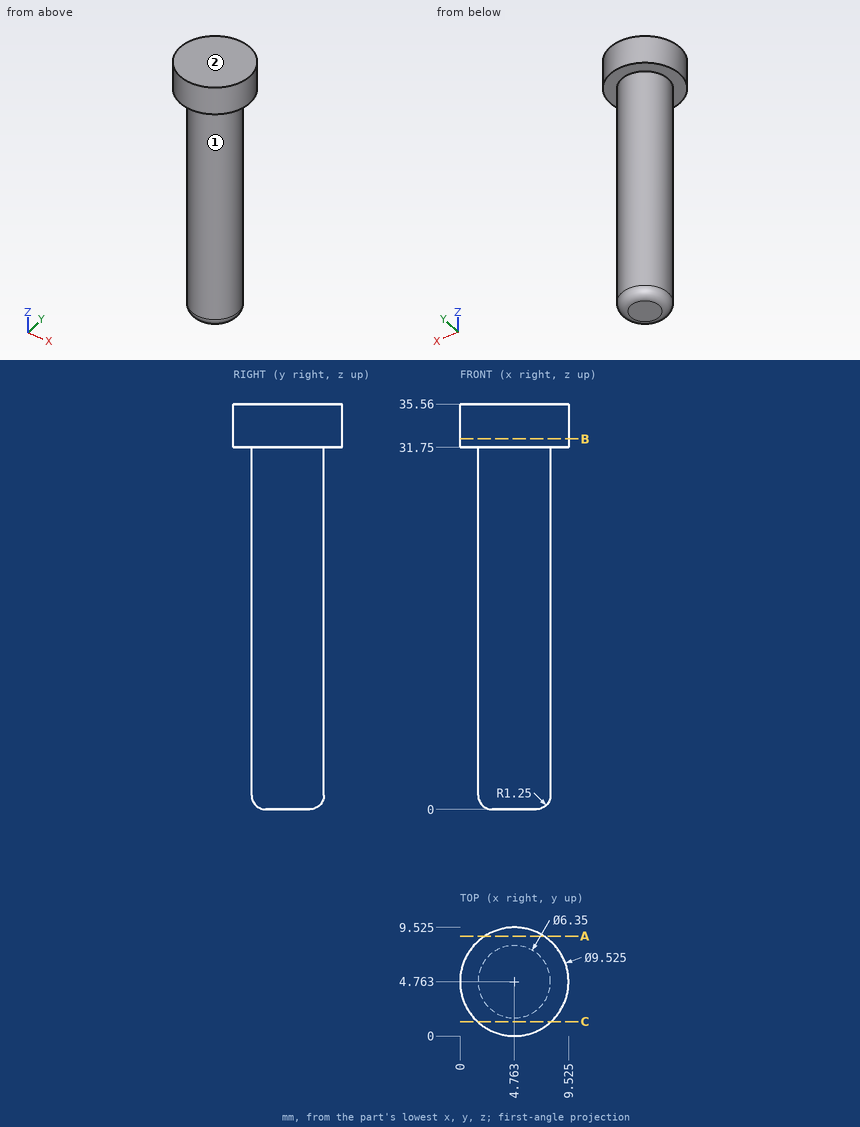
The drawing under review shows one solid part. Ordinate dimensions are in mm from its lowest x, y, z. A direction names the side the tool comes from. Round coordinates to 2 decimals unless told otherwise and drop trailing zeros. Loops run counter-clockwise (first coordinate to the right, second up) from the corner with the lowest first, then second, coordinate; pieces in that order, holes last. Notation, with made-up numbers: (39.25, 82.25) - (73.25, 82.25) arc R30 cw to (73.25, 108.25) - close; hole circle Ø1 at (38, 41.5). An arc over 180 degrees is marked (long way). Use a Markdown table: item, result. Add a question column.
Q1. Machinability: for the marked faces 1 and 2, which of the approach directions +Z, -Z, +X, -X, +Y, -Y give a long, thin tool a straight path to every point of the face, cutting with its end or side? Answer none if there is none.
Q2. Insertion check: pin 1 Ø2 at (x, z) = (5, 13) entering from +Y; pin 2 Ø1 at (x, z) = (5.5, 27) entering from -Y. Each pin has a flat end and moves straight along its axis. Give the tip position at first contact, or say it passes through.
Q3. For probe 1 along Z at (x, y) = (3.25, 1); probe 2 along Y at (x, z) = (4.75, 5); probe 3 along Y at (x, z) = (2.5, 26.5) (1 decimal), list the stretches that pass through material, from the lowest coordinate up.
Q4. Add section C-C (y = 1.25). State the section outline as (x, z) points.
Q5. Add section B-B (z = 32.5). State the section outline as (x, y) points (1 decimal).
Q6. Add section A-A (y = 8.75). State the section outline as (x, z) points.
Worked answers:
| question | item | result |
|---|---|---|
| 1 | face 1 | -Z |
| 1 | face 2 | +Z, +X, -X, +Y, -Y |
| 2 | pin 1 | y = 7.94 |
| 2 | pin 2 | y = 1.6 |
| 3 | probe 1 | 31.75 to 35.56 |
| 3 | probe 2 | 1.59 to 7.94 |
| 3 | probe 3 | 2.5 to 7 |
| 4 | outline | (1.55, 31.75) - (7.98, 31.75) - (7.98, 35.56) - (1.55, 35.56) - close |
| 5 | outline | circle Ø9.5 at (4.8, 4.8) |
| 6 | outline | (2.16, 31.75) - (7.37, 31.75) - (7.37, 35.56) - (2.16, 35.56) - close |
